```python
from build123d import *

# Parameters (mm, degrees)
HEAD_DEPTH     = 15.748
SHANK_SKETCH_R = 7.9375
SHANK_DEPTH    = 82.55
THREAD_END_W   = 38.1
THREAD_END_H   = 0.05


with BuildPart() as part:
    # Head Sketch → Head (new body)
    with BuildSketch(Plane.XY):
        Polygon((0, 13.638168059), (11.811, 6.819084029), (11.811, -6.819084029), (0, -13.638168059), (-11.811, -6.819084029), (-11.811, 6.819084029), align=None)
    extrude(amount=HEAD_DEPTH)

    # Shank Sketch → Shank (add)
    with BuildSketch(Plane.XY):
        Circle(SHANK_SKETCH_R)
    extrude(amount=-SHANK_DEPTH)

    # Sketch3 → Flange (revolve)
    with BuildSketch(Plane(origin=(0, 0, 0), x_dir=(-1, 0, 0), z_dir=(0, 1, 0))):
        with BuildLine():
            Line((-16.891, 0), (0, 0))
            Line((0, 0), (0, 5))
            ThreePointArc((0, 5), (-8.794301894, 3.972903196), (-17.115237243, 0.946897817))
            ThreePointArc((-17.115237243, 0.946897817), (-17.377543373, 0.384780446), (-16.891, 0))
        make_face()
    revolve(axis=Axis((0, 0, 0), (0, 0, 1)))

    # Thread End → Thread Cut (revolve, cut)
    with BuildSketch(Plane(origin=(0, 0, 0), x_dir=(0, 0, -1), z_dir=(1, 0, 0))):
        with Locations((63.5, 7.9125)):
            Rectangle(THREAD_END_W, THREAD_END_H)
    revolve(axis=Axis((0, 0, -21.551935625), (0, 0, -1)), mode=Mode.SUBTRACT)


solid = part.part
```
CAD build for the part. Positions are in the model's coordinates, mm. A direction names the side the tool comes from. Round coordinates to 2 decimals unless told otherwise and drop trailing zeros. Order: outer loops, then holes, each group sorted by start corner. A loop starts at its lowest first (then second) coordinate and runs counter-clockwise, first axis right, second up.
Item 1: Tool access for faces 1 (the face through (-5.99, 10.18, 9.02)), 2 (the face through (5.82, 10.28, 9.02)), 3 (the face through (-4.8, -6.26, -63.77)), 4 (the face through (5.99, -10.18, 9.02)): list every direction of +Z, -Z, +X, -X, +Y, -Y with a clear straight run to the whole face (end or side of a thin tool).
Item 2: Saw through at B-B on z = -6.5. Write the cut outline in (x, y) (1 decimal).
Item 3: Pin check, flat tips, straight feed: pin 1 (1.5 mm diameter, centred on x = 12, y = -8, fed in from +Z); pin 2 (8 mm diameter, centred on x = 10.5, z = -14, fed in from -Y); pin 3 (10.5 mm diameter, centred on y = -2.5, z = 10.5, fed in from +X). Stop position of each tip, or through.
Item 4: Saw through at C-C on z = -66. Write the cut outline in (x, y) (1 decimal), then the cut area to 3 significant figures.
Item 5: Saw through at A-A on y = 0. Write the cut outline in (x, z), then the cut area to 3 significant figures.
Item 6: Probe line 1 along Z through (x, y) = (-8, -1); line 2 along X through (y, z) = (-6, -66.5); line 3 along Y through (x, z) = (-4, -23). List the from-to ranges inside material, lowest first.
Reported:
1. face 1: +Z, -X, +Y
1. face 2: +Z, +X, +Y
1. face 3: -Z
1. face 4: +Z, +X, -Y
2. outline: circle Ø15.9 at (0, 0)
3. pin 1: stops at z = 2.47
3. pin 2: stops at y = -4.56
3. pin 3: stops at x = 11.81
4. outline: circle Ø15.8 at (0, 0)
4. area: 195 mm2
5. outline: (-17.12, 0.95) arc R0.5 ccw to (-16.89, 0) - (-7.94, 0) - (-7.94, -44.45) - (-7.89, -44.45) - (-7.89, -82.55) - (7.89, -82.55) - (7.89, -44.45) - (7.94, -44.45) - (7.94, 0) - (16.89, 0) arc R0.5 ccw to (17.12, 0.95) arc R38.16 ccw to (11.81, 3.13) - (11.81, 15.75) - (-11.81, 15.75) - (-11.81, 3.13) arc R38.16 ccw to start
5. area: 1,700 mm2
6. line 1: z = 0 to 15.75
6. line 2: x = -5.12 to 5.12
6. line 3: y = -6.86 to 6.86
